```python
from build123d import *

# Parameters (mm, degrees)
SKETCH2_W                                  = 28.5
SKETCH2_H                                  = 93
SKETCH2_R                                  = 10.75
BOSS_EXTRUDE1_DEPTH                        = 2.3
BOSS_EXTRUDE2_DEPTH                        = 2.9
CBORE_FOR_M2_5_PAN_HEAD_SCREW1_D           = 2.9
CBORE_FOR_M2_5_PAN_HEAD_SCREW1_DEPTH       = 8
CBORE_FOR_M2_5_PAN_HEAD_SCREW1_CBORE_D     = 4.4
CBORE_FOR_M2_5_PAN_HEAD_SCREW1_CBORE_DEPTH = 2.1
CBORE_FOR_M2_5_PAN_HEAD_SCREW1_TIP         = 0.871247898
CHAMFER1_SIZE                              = 2
CHAMFER2_SIZE                              = 0.5


with BuildPart() as part:
    # Sketch2 → Boss-Extrude1 (new body)
    with BuildSketch(Plane.XY):
        with Locations((0, -35.25)):
            Rectangle(SKETCH2_W, SKETCH2_H)
        Circle(SKETCH2_R, mode=Mode.SUBTRACT)
        with Locations(Location((0, -70.5, 0), (0, 0, 180))):
            Circle(SKETCH2_R, mode=Mode.SUBTRACT)
    extrude(amount=BOSS_EXTRUDE1_DEPTH)

    # Sketch3 → Boss-Extrude2 (add)
    with BuildSketch(Plane(origin=(0, 0, 0), x_dir=(-1, 0, 0), z_dir=(0, 0, -1))):
        with BuildLine():
            Line((7.75, 11.25), (7.75, 8))
            ThreePointArc((7.75, 8), (8.701902961, 5.701902961), (11, 4.75))
            Line((11, 4.75), (14.25, 4.75))
            Line((14.25, 4.75), (14.25, 11.25))
            Line((14.25, 11.25), (7.75, 11.25))
        make_face()
        with BuildLine():
            Line((11, -41.75), (14.25, -41.75))
            Line((14.25, -41.75), (14.25, -28.75))
            Line((14.25, -28.75), (11, -28.75))
            ThreePointArc((11, -28.75), (8.701902961, -29.701902961), (7.75, -32))
            Line((7.75, -32), (7.75, -38.5))
            ThreePointArc((7.75, -38.5), (8.701902961, -40.798097039), (11, -41.75))
        make_face()
        with BuildLine():
            Line((14.25, -81.75), (7.75, -81.75))
            Line((7.75, -81.75), (7.75, -78.5))
            ThreePointArc((7.75, -78.5), (8.701902961, -76.201902961), (11, -75.25))
            Line((11, -75.25), (14.25, -75.25))
            Line((14.25, -75.25), (14.25, -81.75))
        make_face()
        with BuildLine():
            Line((-14.25, 11.25), (-7.75, 11.25))
            Line((-7.75, 11.25), (-7.75, 8))
            ThreePointArc((-7.75, 8), (-8.701902961, 5.701902961), (-11, 4.75))
            Line((-11, 4.75), (-14.25, 4.75))
            Line((-14.25, 4.75), (-14.25, 11.25))
        make_face()
        with BuildLine():
            Line((-7.75, -38.5), (-7.75, -32))
            ThreePointArc((-7.75, -32), (-8.701902961, -29.701902961), (-11, -28.75))
            Line((-11, -28.75), (-14.25, -28.75))
            Line((-14.25, -28.75), (-14.25, -41.75))
            Line((-14.25, -41.75), (-11, -41.75))
            ThreePointArc((-11, -41.75), (-8.701902961, -40.798097039), (-7.75, -38.5))
        make_face()
        with BuildLine():
            Line((-7.75, -81.75), (-7.75, -78.5))
            ThreePointArc((-7.75, -78.5), (-8.701902961, -76.201902961), (-11, -75.25))
            Line((-11, -75.25), (-14.25, -75.25))
            Line((-14.25, -75.25), (-14.25, -81.75))
            Line((-14.25, -81.75), (-7.75, -81.75))
        make_face()
    extrude(amount=BOSS_EXTRUDE2_DEPTH)

    # CBORE for M2.5 Pan Head Screw1
    with Locations(Plane.XY.offset(2.3)):
        with Locations((-11, 8), (11, 8), (11, -32), (-11, -32), (-11, -38.5), (11, -38.5), (11, -78.5), (-11, -78.5)):
            CounterBoreHole(CBORE_FOR_M2_5_PAN_HEAD_SCREW1_D / 2, CBORE_FOR_M2_5_PAN_HEAD_SCREW1_CBORE_D / 2, CBORE_FOR_M2_5_PAN_HEAD_SCREW1_CBORE_DEPTH, depth=CBORE_FOR_M2_5_PAN_HEAD_SCREW1_DEPTH)
            with Locations((0, 0, -(CBORE_FOR_M2_5_PAN_HEAD_SCREW1_DEPTH + CBORE_FOR_M2_5_PAN_HEAD_SCREW1_TIP / 2))):  # 118° drill point
                Cone(0, CBORE_FOR_M2_5_PAN_HEAD_SCREW1_D / 2, CBORE_FOR_M2_5_PAN_HEAD_SCREW1_TIP, mode=Mode.SUBTRACT)

    # Chamfer1
    chamfer1_edges = [part.edges().sort_by_distance(p)[0] for p in [
        (-14.25, 11.25, -0.3),
        (14.25, 11.25, -0.3),
        (14.25, -81.75, -0.3),
        (-14.25, -81.75, -0.3),
    ]]
    chamfer(chamfer1_edges, length=CHAMFER1_SIZE)

    # Chamfer2
    chamfer2_edges = [part.edges().sort_by_distance(p)[0] for p in [
        (0, -81.75, 2.3),
        (-14.25, -35.25, 2.3),
        (14.25, -35.25, 2.3),
        (0, 11.25, 2.3),
        (-13.25, 10.25, 2.3),
        (13.25, 10.25, 2.3),
        (13.25, -80.75, 2.3),
        (-13.25, -80.75, 2.3),
    ]]
    chamfer(chamfer2_edges, length=CHAMFER2_SIZE - 0.0001)  # a hair under: the kernel refuses the full size


solid = part.part
```
CAD build for the part. Positions are in the model's coordinates, mm. A direction names the side the tool comes from. Round coordinates to 2 decimals unless told otherwise and drop trailing zeros. Loops run counter-clockwise (first coordinate to the right, second up) from the corner with the lowest first, then second, coordinate; pieces in that order, holes last. Notation, with made-up numbers: M -31.5,77 L -8.5,77 A24 cw -8.5,93 Z; hole C 6.25,-30.75 d4. An arc over 180 degrees is marked long. Use a Markdown table: item, result. Add a question column.
(1) Cut at B-B (y = -70.5). Give the cut face in (x, z).
(2) Pull direction X, two halves, no side cores. Call faces 1 (the face through (-9.817, 9.855, 1.265)), 2 (the face through (-11.7, 9.5, -2.9)), 3 (the face through (-9.85, 7.12, -1.37)): +X half, -X half, draft (parallel to the pull), parting line (faces both ways), or undercut.
(3) Flat gauge pin, fed straight in: pin 1 (4 mm diameter, centred on x = -11, y = -38.5, fed in from +Z). Where does the tip first touch, or does it go through?
(4) Which spindle directions (+Z, -Z, +X, -X, +Y, -Y) get a long thin tool onto all of the face, cutting with end or side? Do faces 4 (the face through (-12, -40, 0.2)), 5 (the face through (8.677, 5.727, -1.43)), 6 (the face through (13, 4.75, -1)), 7 (the face through (7.75, -35, -1)). Say none if no direction does.
(5) Cut at A-A (z = 1). State how many separate pieces and enclosed holes the cut face has, and give its area (3 significant figures).
(6) Cut at D-D (y = -48). Give the cut face in (x, z).
(7) Drill centre lines: line 1 (Y direction, x = 0, z = 0.55); line 2 (Y direction, x = -8, z = -2.55); line 3 (X direction, y = 0, z = 0.85). Where is each one in solid material? Low to high.
Geometry says:
| question | item | result |
|---|---|---|
| 1 | outline | M -14.25,0 L -10.75,0 L -10.75,2.3 L -13.75,2.3 L -14.25,1.8 Z; M 10.75,0 L 14.25,0 L 14.25,1.8 L 13.75,2.3 L 10.75,2.3 Z |
| 2 | face 1 | undercut |
| 2 | face 2 | draft |
| 2 | face 3 | undercut |
| 3 | pin 1 | stops at z = 0.2 |
| 4 | face 4 | +Z |
| 4 | face 5 | -Z |
| 4 | face 6 | -Z, +X, -X |
| 4 | face 7 | -Z, +Y, -Y |
| 5 | separate pieces | 1 |
| 5 | enclosed holes | 10 |
| 5 | area | 1,790 mm² |
| 6 | outline | M -14.25,0 L 14.25,0 L 14.25,1.8 L 13.75,2.3 L -13.75,2.3 L -14.25,1.8 Z |
| 7 | line 1 | y = -81.75 to -81.25, -59.75 to -10.75, 10.75 to 11.25 |
| 7 | line 2 | y = -81.75 to -77.25, -39.75 to -30.75, 6.75 to 11.25 |
| 7 | line 3 | x = -14.25 to -10.75, 10.75 to 14.25 |
